Design review of the part shown in the three views and the two pictorial views. Dimensions are in mm from the part's minimum x, y and z. Round coordinates to 2 decimals unless told otherwise and drop trailing zeros. Loops run counter-clockwise (first coordinate to the right, second up) from the corner with the lowest first, then second, coordinate; pieces in that order, holes last. Notation, with made-up numbers: (76.5, -13) -> (105.5, -13) arc R6 ccw to (105.5, -4) -> close; hole circle Ø6 at (23.5, -18.5). An arc over 180 degrees is marked (long way). Use CSV: the item, a comma, the result in double quotes. Start each with the question number.
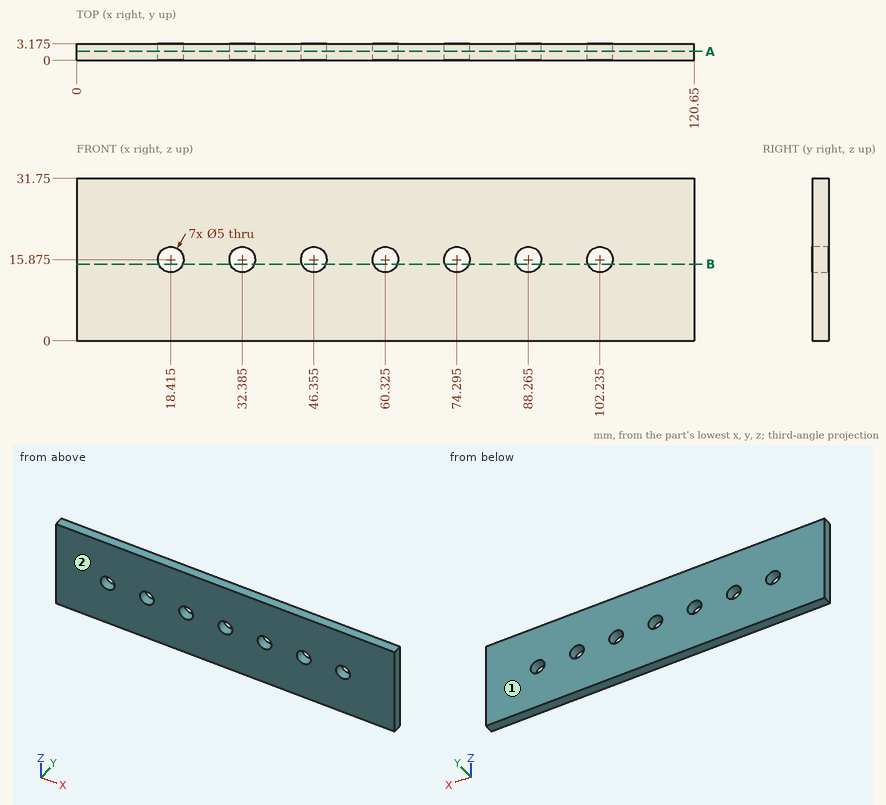
1. The part is to be moulded in two halves that separate along Y. For the marked faces 1 and 2, say which applies: pulls with the +Y half, pulls with the -Y half, needs draft (parallel to the pull), parting line crosses it, or undercut.
2. Take a section at B-B, the plane z = 15. Count the separate pieces of the cut face and the enclosed holes in it, then the cut area to 3 significant figures.
3. For line 1 along Z through (x, y) = (18, 2.9); line 2 along Z through (x, y) = (47, 1.4), list the stretches that pass through material, from the lowest coordinate up. Write a range as from..to.
4. Take a section at A-A, the plane y = 1.75. Give the boundary of the cut face in (x, z) (3 decimals), then the cut area to 3 significant figures.
Results:
1,face 1,"pulls with the +Y half"
1,face 2,"pulls with the -Y half"
2,separate pieces,"8"
2,enclosed holes,"0"
2,area,"279 mm²"
3,line 1,"0..13.41, 18.34..31.75"
3,line 2,"0..13.46, 18.29..31.75"
4,outline,"(0, 0) -> (120.65, 0) -> (120.65, 31.75) -> (0, 31.75) -> close; hole circle Ø5 at (18.415, 15.875); hole circle Ø5 at (32.385, 15.875); hole circle Ø5 at (46.355, 15.875); hole circle Ø5 at (60.325, 15.875); hole circle Ø5 at (74.295, 15.875); hole circle Ø5 at (88.265, 15.875); hole circle Ø5 at (102.235, 15.875)"
4,area,"3,690 mm²"
